The model under review builds one solid part; all positions refer to its coordinate system, in mm. Face numbers are marked on the shaded views. Coordinates: 2 decimals unless noted, no trailing zeros. Loops run counter-clockwise (first coordinate to the right, second up) from the corner with the lowest first, then second, coordinate; pieces in that order, holes last. Notation, with made-up numbers: M -2.5,27 L 53.5,27 A38 cw 53.5,65 Z; hole C 61,28 d3. An arc over 180 degrees is marked long. Use CSV: the item, a comma, the result in double quotes. Start each with the question number.
1. Add section A-A, the plane z = 0. Write out the cut boundary in (x, y).
2. For L1, parallel to Z at x = 0, y = -0.8; L2, parallel to X at y = 1.2, z = -0.5; L3, parallel to Z at x = -4.75, y = 0.9, list the stretches that pass through material, from the lowest coordinate up.
3. Add section B-B, the plane y = -0.75. Write out the cut boundary in (x, z), then the cut area to 3 significant figures.
4. Clearance check with a flat-ended pin moving along its axis: P1, Ø2, axis at y = -1.5, z = 3, coming from the +X side. State where the tip first meets the part, or that it passes through.
5. Add section D-D, the plane x = 6.5. Write out the cut boundary in (y, z), then the cut area to 3 significant figures.
6. Add section C-C, the plane x = 0. Write out the cut boundary in (y, z), then the cut area to 3 significant figures.
7. Draft analysis for pull direction X (two halves, no side actions). For the marked faces 1, 2 and 3, state which applies: +X half, -X half, draft (parallel to the pull), parting line (faces both ways), or undercut.
from build123d import *

# Parameters (mm, degrees)
F1_DEPTH    = 2
F2_T1_DEPTH = 4


# Not quite as in the source:
# - a fillet or chamfer that OpenCascade refuses, or shapes differently, is made with other operations: its cross-section is extruded or revolved along the edge and cut away or added


with BuildPart() as f1:
    # F0 (on Front) → F1 (new body, symmetric)
    with BuildSketch(Plane.XZ):
        with BuildLine():
            ThreePointArc((-4.7906232606, -7.6190503854), (-2.4928444127, -8.6478741165), (0, -9))
            ThreePointArc((0, -9), (2.4928444127, -8.6478741165), (4.7906232606, -7.6190503854))
            Line((4.7906232606, -7.6190503854), (5.6568542495, -8.4852813742))
            Line((5.6568542495, -8.4852813742), (8.4852813742, -5.6568542495))
            Line((8.4852813742, -5.6568542495), (7.6190503854, -4.7906232606))
            ThreePointArc((7.6190503854, -4.7906232606), (0, 9), (-7.6190503854, -4.7906232606))
            Line((-7.6190503854, -4.7906232606), (-8.4852813742, -5.6568542495))
            Line((-8.4852813742, -5.6568542495), (-5.6568542495, -8.4852813742))
            Line((-5.6568542495, -8.4852813742), (-4.7906232606, -7.6190503854))
        make_face()
        with BuildLine():
            ThreePointArc((0, -6), (-4.2426406871, 4.2426406871), (6, 0))
            ThreePointArc((6, 0), (4.2426406871, -4.2426406871), (0, -6))
        make_face(mode=Mode.SUBTRACT)
    extrude(amount=F1_DEPTH, both=True)

    # F2: fillet of radius 5 on 4 edges, made by hand

    # F2_s2 → F2_t1 (join)
    with BuildSketch(Plane.XZ.offset(-2)):
        with BuildLine():
            ThreePointArc((8.5560838448, -2.7916714064), (8.3109896839, -4.2190810375), (8.4852813742, -5.6568542495))
            Line((8.4852813742, -5.6568542495), (7.6190503854, -4.7906232606))
            ThreePointArc((7.6190503854, -4.7906232606), (8.149091604, -3.8199877003), (8.5560838448, -2.7916714064))
        make_face()
        with BuildLine():
            ThreePointArc((5.6568542495, -8.4852813742), (4.2190810375, -8.3109896839), (2.7916714064, -8.5560838448))
            ThreePointArc((2.7916714064, -8.5560838448), (3.8199877003, -8.149091604), (4.7906232606, -7.6190503854))
            Line((4.7906232606, -7.6190503854), (5.6568542495, -8.4852813742))
        make_face()
        with BuildLine():
            ThreePointArc((-2.7916714064, -8.5560838448), (-4.2190810375, -8.3109896839), (-5.6568542495, -8.4852813742))
            Line((-5.6568542495, -8.4852813742), (-4.7906232606, -7.6190503854))
            ThreePointArc((-4.7906232606, -7.6190503854), (-3.8199877003, -8.149091604), (-2.7916714064, -8.5560838448))
        make_face()
        with BuildLine():
            ThreePointArc((-8.4852813742, -5.6568542495), (-8.3109896839, -4.2190810375), (-8.5560838448, -2.7916714064))
            ThreePointArc((-8.5560838448, -2.7916714064), (-8.149091604, -3.8199877003), (-7.6190503854, -4.7906232606))
            Line((-7.6190503854, -4.7906232606), (-8.4852813742, -5.6568542495))
        make_face()
    extrude(amount=F2_T1_DEPTH)


solid = f1.part
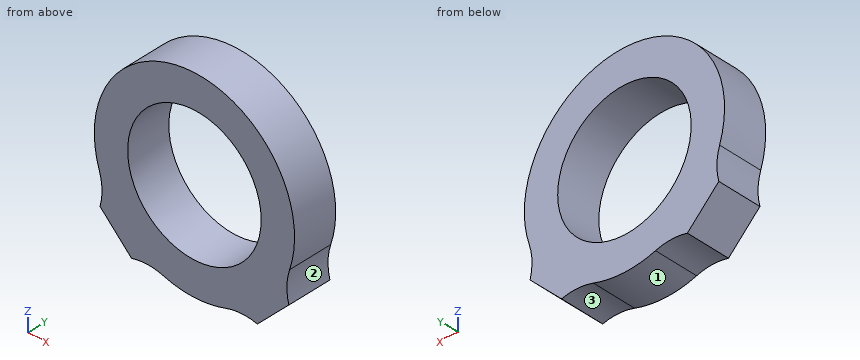
Computed:
1,outline,"M -9,-2 L -6,-2 L -6,2 L -9,2 Z; M 6,-2 L 9,-2 L 9,2 L 6,2 Z"
2,L1,"z = -9 to -6, 6 to 9"
2,L2,"x = -8.99 to -5.98, 5.98 to 8.99"
2,L3,"z = -8.33 to -3.67, 3.67 to 7.64"
3,outline,"M -8.56,-2.79 A5 cw -8.49,-5.66 L -5.66,-8.49 A5 cw -2.79,-8.56 A9 ccw 2.79,-8.56 A5 cw 5.66,-8.49 L 8.49,-5.66 A5 cw 8.56,-2.79 A9 ccw long Z; hole C 0,0 d12"
3,area,"153 mm^2"
4,P1,"stops at x = 8.77"
5,outline,"M -2,-7.64 L 2,-7.64 L 2,6.22 L -2,6.22 Z"
5,area,"55.5 mm^2"
6,outline,"M -2,-9 L 2,-9 L 2,-6 L -2,-6 Z; M -2,6 L 2,6 L 2,9 L -2,9 Z"
6,area,"24.0 mm^2"
7,face 1,"parting line"
7,face 2,"+X half"
7,face 3,"undercut"
